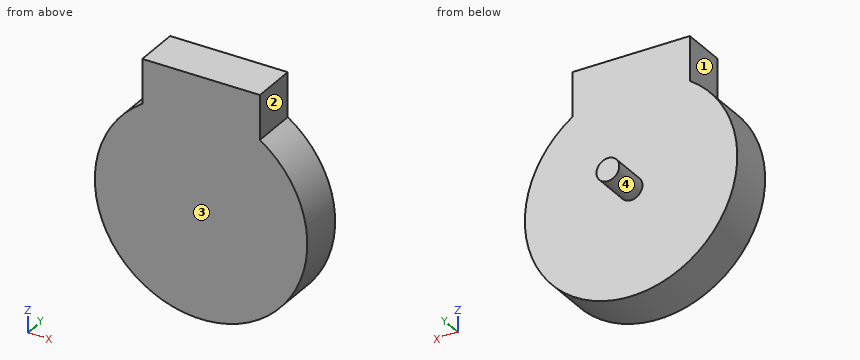
Autodesk Inventor part; units mm, degrees
ref_plane "YZ Plane" through (0, 0, 0) normal (1, 0, 0) x (0, 1, 0)
ref_plane "XZ Plane" through (0, 0, 0) normal (0, 1, 0) x (-1, 0, 0)
ref_plane "XY Plane" through (0, 0, 0) normal (0, 0, 1) x (1, 0, 0)
sketch "Sketch1" plane through (0, 0, 0) normal (0, 1, 0) x (-1, 0, 0)
  circle A0 centre (0, 0) radius 28
  dimension "d0" = 56
extrude "Extrusion1" add sketch "Sketch1" along normal blind 12
sketch "Sketch3" plane through (0, 0, 0) normal (0, 0, 1) x (1, 0, 0)
  line L0 (0, 11.8294) -> (-15.4991, 12)
  line L1 (28, 12) -> (-28, 12)
  line L2 (-15.4991, 12) -> (-15.4991, -22.0673)
  line L3 (-28, 0) -> (28, 0)
  line L4 (-15.4991, 12) -> (15.5009, 12)
  line L5 (15.5009, 12) -> (15.5009, 0)
  line L6 (15.5009, 0) -> (-15.4991, 0)
  line L7 (-15.4991, 0) -> (-15.4991, 12)
  point P0 (0, 0)
  dimension "d5" = 15.5
  dimension "d6" = 31
extrude "Extrusion2" add sketch "Sketch3" along normal blind 35
sketch "Sketch4" plane through (0, 12, 0) normal (0, 1, 0) x (1, 0, 0)
  arc A0 (15.5009, -23.3178) -> (-15.4991, -23.3191) centre (0, 0) ccw
  circle A1 centre (0, 0) radius 3
  dimension "d9" = 6
extrude "Extrusion3" add sketch "Sketch4" along normal blind 10
properties part number "Encoder model"
Verification items for the finished model (mm, model axes). Face numbers are marked on the shaded views. A direction names the side the tool comes from. Give positions to 0.01 mm unless a question says otherwise; leave off trailing zeros. Loops run counter-clockwise (first coordinate to the right, second up) from the corner with the lowest first, then second, coordinate; pieces in that order, holes last.
1. Section check A-A, the plane z = 0. Enter the section's corners in (x, y).
2. Section check B-B, the plane x = 0. Enter the section's corners in (y, z).
3. Section check C-C, the plane y = 5.25. Enter the section's corners in (x, z), then the cut area to 3 significant figures.
4. Thickness scan on line 1 (Y direction, x = 9, z = -19.5); line 2 (Z direction, x = -20, y = 7); line 3 (X direction, y = 10.5, z = 6). Record the ranges inside material, lowest first.
5. Set-up check for the marked faces 1, 2, 3 and 4: record each of +Z, -Z, +X, -X, +Y, -Y from which the full face is reachable in a straight line by a thin tool's end or side.
6. Go/stop test with flat-tipped pins: pin 1 Ø6 at (y, z) = (6, 30) entering from -X; pin 2 Ø1.5 at (x, z) = (-7, -16.5) entering from +Y; pin 3 Ø3.5 at (y, z) = (4, 30.5) entering from +X. Record where each tip stops, or that it passes through.
7. Section check D-D, the plane z = 24.5. Enter the section's corners in (x, y), then the cut area to 3 significant figures.
Geometry says:
1. outline: (-28, 0) - (28, 0) - (28, 12) - (3, 12) - (3, 22) - (-3, 22) - (-3, 12) - (-28, 12) - close
2. outline: (0, -28) - (12, -28) - (12, -3) - (22, -3) - (22, 3) - (12, 3) - (12, 35) - (0, 35) - close
3. outline: (-15.5, 23.32) arc R28 ccw (long way) to (15.5, 23.32) - (15.5, 35) - (-15.5, 35) - close
3. area: 2,730 mm2
4. line 1: y = 0 to 12
4. line 2: z = -19.6 to 19.6
4. line 3: x = -27.35 to 27.35
5. face 1: +Z, -X, +Y, -Y
5. face 2: +Z, +X, +Y, -Y
5. face 3: +Z, -Z, +X, -X, -Y
5. face 4: +Y
6. pin 1: stops at x = -15.5
6. pin 2: stops at y = 12
6. pin 3: stops at x = 15.5
7. outline: (-15.5, 0) - (15.5, 0) - (15.5, 12) - (-15.5, 12) - close
7. area: 372 mm2
